For this review, take the finished solid that the model builds, in its own axes (mm). A direction names the side the tool comes from. Give positions to 0.01 mm unless a question says otherwise; leave off trailing zeros. Order: outer loops, then holes, each group sorted by start corner. A loop starts at its lowest first (then second) coordinate and runs counter-clockwise, first axis right, second up.
Item 1: The part is to be moulded in two halves that separate along X. For faces 3 (the cylindrical face through (-2.17, 9.76, -14.55)), 4 (the flat face through (4, 4, 0)), 5 (the flat face through (0, 0, -20)), say which applies: released by +X, released by -X, zero draft, split by the parting line, or undercut.
Item 2: Machinability: for faces 1 (the flat face through (0, 0, -30)), 2 (the cylindrical face through (-1.08, 4.88, -10.39)), which of the approach directions +Z, -Z, +X, -X, +Y, -Y give a long, thin tool a straight path to every point of the face, cutting with its end or side? Answer none if there is none.
Item 3: Consider section C-C (z = -14). Give the boundary of the cut face in (x, y).
Item 4: For probe 1 along Y at (x, z) = (0, -14.5); probe 2 along X at (y, z) = (2, -19), list the stretches that pass through material, from the lowest coordinate up.
Item 5: Consider section A-A (y = 0). Give the boundary of the cut face in (x, z).
Item 6: For P1, Ø6, axis at x = 4.5, z = -8, coming from the -Y side; P2, Ø3, axis at x = 3, z = -10, coming from the +Y side; P3, Ø2, axis at y = 5, z = -18, coming from the -X side, all flat-tipped, find the tip position at first contact; note any pin that passes through.
```python
from build123d import *

# Parameters (mm, degrees)
F2_SIZE = 1
F3_SIZE = 0.5


with BuildPart() as f1:
    # F0 (on Front) → F1 (revolve)
    with BuildSketch(Plane.XZ):
        Polygon((0, -20), (0, -30), (10, -30), (10, 0), (5, 0), (5, -20), align=None)
    revolve(axis=Axis((0, 0, -25), (0, 0, -1)))

    # F2
    f2_edges = [f1.edges().sort_by_distance(p)[0] for p in [
        (-10, 0, -30),
    ]]
    chamfer(f2_edges, length=F2_SIZE)

    # F3
    f3_edges = [f1.edges().sort_by_distance(p)[0] for p in [
        (-10, 0, 0),
        (-5, 0, 0),
    ]]
    chamfer(f3_edges, length=F3_SIZE)


solid = f1.part
```
Resolved:
1. face 3: split by the parting line
1. face 4: zero draft
1. face 5: undercut
2. face 1: -Z, +X, -X, +Y, -Y
2. face 2: +Z
3. outline: circle Ø20 at (0, 0); hole circle Ø10 at (0, 0)
4. probe 1: y = -10 to -5, 5 to 10
4. probe 2: x = -9.8 to -4.58, 4.58 to 9.8
5. outline: (-10, -29) - (-9, -30) - (9, -30) - (10, -29) - (10, -0.5) - (9.5, 0) - (5.5, 0) - (5, -0.5) - (5, -20) - (-5, -20) - (-5, -0.5) - (-5.5, 0) - (-9.5, 0) - (-10, -0.5) - close
6. P1: stops at y = -9.89
6. P2: stops at y = 9.89
6. P3: stops at x = -9.17
